Work out the finished part from the listing and answer in its coordinate system (mm). A direction names the side the tool comes from. Round coordinates to 2 decimals unless told otherwise and drop trailing zeros. Write each loop counter-clockwise with the first axis right and the second up, starting at its lowest first coordinate (ties: lowest second). Pieces come first, ordered by that corner, then holes. Notation, with made-up numbers: M 27.5,23.5 L 80.5,23.5 A18 ccw 80.5,45.5 Z; hole C 47.25,17 d8. An arc over 180 degrees is marked long. One line per item, written item: value. Start each with the question number.
Q1. Find section A-A (x = 0). Write down the section's boundary in (y, z), and give its area (3 significant figures).
Q2. Find section D-D (x = 20). Write down the section's boundary in (y, z).
Q3. Consider probe 1 along Y at (x, z) = (0, 1.25); probe 2 along Y at (x, z) = (20, -3.2); probe 3 along Y at (x, z) = (7, 1.5). Determine where each line is inside the solid, lowest interval first.
Q4. Given pin 1 Ø1.8 at (x, y) = (18.5, 11) entering from -Z; pin 2 Ø1.9 at (x, y) = (0, 0) entering from +Z; pin 3 Ø4.5 at (x, y) = (-11.5, -3) entering from +Z, each flat-ended and moving along its own axis, determine where each tip first touches the part or whether it passes through.
Q5. Find section C-C (y = -26). Write down the section's boundary in (x, z), and give its area (3 significant figures).
Q6. The mould has two halves that part along X. Classify faces 1 (the flat face through (-13, -4, -2)), 2 (the flat face through (-25, -8, 0)), 3 (the flat face through (0, -24, 3)): released by +X, released by -X, zero draft, split by the parting line, or undercut.
Q7. A tool of negligible diameter and unlimited length cuts with its end or side. For faces 4 (the cylindrical face through (-17.476, -17.907, -0.451)), 5 (the flat face through (25, -8, 0)), 6 (the cylindrical face through (-23, 9.9, -3.5)), 7 (the flat face through (-0.2, -17, -1.5)), from which of +Z, -Z, +X, -X, +Y, -Y can it reach the whole face along a straight path? Write none if from no direction.
Q8. Find section B-B (z = 1.25). Write down the section's boundary in (x, y), and give its area (3 significant figures).
from build123d import *

# Parameters (mm, degrees)
F0_R     = 1.6
F1_DEPTH = 3
F2_DEPTH = 3
F3_W     = 50
F3_H     = 46
F4_DEPTH = 6
F6_DEPTH = 1
F7_DEPTH = 1
F8_R     = 3
F9_DEPTH = 1


with BuildPart() as f1:
    # F0 (on Top) → F1 (new body)
    with BuildSketch(Plane.XY):
        with BuildLine():
            ThreePointArc((-8.4251758935, 3.1648714292), (-1.6083247431, -8.8551279788), (9, 0))
            ThreePointArc((9, 0), (8.8551279788, 1.6083247431), (8.4251758935, 3.1648714292))
            ThreePointArc((8.4251758935, 3.1648714292), (0, 9), (-8.4251758935, 3.1648714292))
        make_face()
        Circle(F0_R, mode=Mode.SUBTRACT)
        with BuildLine():
            ThreePointArc((8.4251758935, 3.1648714292), (8.8551279788, 1.6083247431), (9, 0))
            ThreePointArc((9, 0), (-1.6083247431, -8.8551279788), (-8.4251758935, 3.1648714292))
            Line((-8.4251758935, 3.1648714292), (-14.4767774381, -12.9450428569))
            ThreePointArc((-14.4767774381, -12.9450428569), (-14.1346449317, -15.7080879033), (-11.6683854736, -17))
            Line((-11.6683854736, -17), (0, -17))
            Line((0, -17), (11.6683854736, -17))
            ThreePointArc((11.6683854736, -17), (14.1346449317, -15.7080879033), (14.4767774381, -12.9450428569))
            Line((14.4767774381, -12.9450428569), (8.4251758935, 3.1648714292))
        make_face()
    extrude(amount=-F1_DEPTH)

    # F0 (on Top) → F2 (join)
    with BuildSketch(Plane.XY):
        with BuildLine():
            ThreePointArc((-8.4251758935, 3.1648714292), (-1.6083247431, -8.8551279788), (9, 0))
            ThreePointArc((9, 0), (8.8551279788, 1.6083247431), (8.4251758935, 3.1648714292))
            ThreePointArc((8.4251758935, 3.1648714292), (0, 9), (-8.4251758935, 3.1648714292))
        make_face()
        Circle(F0_R, mode=Mode.SUBTRACT)
    extrude(amount=F2_DEPTH)



with BuildPart() as f4:
    # F3 (on face) → F4 (new body, through all)
    with BuildSketch(Plane(origin=(0, 0, -3), x_dir=(1, 0, 0), z_dir=(0, 0, -1))):
        with Locations((0, 8)):
            Rectangle(F3_W, F3_H)
        with BuildLine():
            Line((-12.1696985129, -4.5714809533), (-18.2213000575, 11.5384333329))
            ThreePointArc((-18.2213000575, 11.5384333329), (-17.4229908758, 17.985538441), (-11.6683854736, 21))
            Line((-11.6683854736, 21), (11.6683854736, 21))
            ThreePointArc((11.6683854736, 21), (17.4229908758, 17.985538441), (18.2213000575, 11.5384333329))
            Line((18.2213000575, 11.5384333329), (12.1696985129, -4.5714809533))
            ThreePointArc((12.1696985129, -4.5714809533), (0, -13), (-12.1696985129, -4.5714809533))
        make_face(mode=Mode.SUBTRACT)
    extrude(amount=-F4_DEPTH)


with BuildPart() as f1_1:
    add(f1.part)

    add(f4.part)  # F6 merges F4
    # F5 (on face) → F6 (join)
    with BuildSketch(Plane(origin=(0, 0, -3), x_dir=(1, 0, 0), z_dir=(0, 0, -1))):
        with BuildLine():
            Line((-10.2463335535, 1.683216071), (-12.3562478397, 7.3))
            ThreePointArc((-12.3562478397, 7.3), (-13.5252043873, 4.7244339283), (-16.100770459, 5.8933904759))
            Line((-16.100770459, 5.8933904759), (-13.9908561729, 0.2766065469))
            ThreePointArc((-13.9908561729, 0.2766065469), (-12.8218996253, 2.8521726186), (-10.2463335535, 1.683216071))
        make_face()
        with BuildLine():
            ThreePointArc((-3, 21), (-1, 19), (-3, 17))
            Line((-3, 17), (3, 17))
            ThreePointArc((3, 17), (1, 19), (3, 21))
            Line((3, 21), (-3, 21))
        make_face()
        with BuildLine():
            Line((12.3562478397, 7.3), (10.2463335535, 1.683216071))
            ThreePointArc((10.2463335535, 1.683216071), (12.8218996253, 2.8521726186), (13.9908561729, 0.2766065469))
            Line((13.9908561729, 0.2766065469), (16.100770459, 5.8933904759))
            ThreePointArc((16.100770459, 5.8933904759), (13.5252043873, 4.7244339283), (12.3562478397, 7.3))
        make_face()
    extrude(amount=-F6_DEPTH)

    # F7 (add): a face of the model
    f7_faces = [f1_1.faces().sort_by_distance(p)[0] for p in [
        (0, -8.3665022997, -3),
    ]]
    extrude(f7_faces, amount=F7_DEPTH)

    # F8 (on face) → F9 (cut)
    with BuildSketch(Plane(origin=(0, 0, -4), x_dir=(1, 0, 0), z_dir=(0, 0, -1))):
        with Locations((-20, 26)):
            Circle(F8_R)
        with Locations((20, 26)):
            Circle(F8_R)
        with Locations((20, -10)):
            Circle(F8_R)
        with Locations((-20, -10)):
            Circle(F8_R)
    extrude(amount=-F9_DEPTH, mode=Mode.SUBTRACT)


solid = f1_1.part
The answers:
1. outline: M -31,-4 L -1.6,-4 L -1.6,3 L -9,3 L -9,0 L -17,0 L -17,-2 L -21,-2 L -21,3 L -31,3 Z; M 1.6,-4 L 9,-4 L 9,3 L 1.6,3 Z; M 13,-4 L 15,-4 L 15,3 L 13,3 Z
1. area: 228 mm2
2. outline: M -31,-4 L -29,-4 L -29,-3 L -23,-3 L -23,-4 L 7,-4 L 7,-3 L 13,-3 L 13,-4 L 15,-4 L 15,3 L -31,3 Z
3. probe 1: -31 to -21, -9 to -1.6, 1.6 to 9, 13 to 15
3. probe 2: -31 to -29, -23 to 7, 13 to 15
3. probe 3: -31 to -21, -5.66 to 5.66, 10.95 to 15
4. pin 1: z = -3
4. pin 2: through
4. pin 3: z = 0
5. outline: M -25,-4 L -23,-4 L -23,-3 L -17,-3 L -17,-4 L 17,-4 L 17,-3 L 23,-3 L 23,-4 L 25,-4 L 25,3 L -25,3 Z
5. area: 338 mm2
6. face 1: undercut
6. face 2: released by -X
6. face 3: zero draft
7. face 4: +Z, -Z
7. face 5: +Z, -Z, +X, +Y, -Y
7. face 6: -Z
7. face 7: +Z
8. outline: M -25,-31 L 25,-31 L 25,15 L -25,15 Z; C 0,0 d18; hole M -18.22,-11.54 A7 ccw -11.67,-21 L 11.67,-21 A7 ccw 18.22,-11.54 L 12.17,4.57 A13 ccw -12.17,4.57 Z; hole C 0,0 d3.2
8. area: 1,580 mm2
